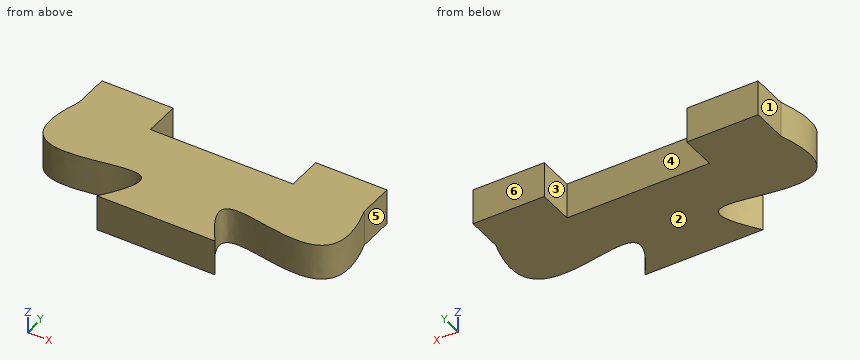
```python
from build123d import *

# Parameters (mm, degrees)
SKETCH1_W           = 6.35
SKETCH1_H           = 3.175
BOSS_EXTRUDE1_DEPTH = 3.175


with BuildPart() as part:
    # Sketch1 → Boss-Extrude1 (new body)
    with BuildSketch(Plane.XY):
        with Locations((-63.39715008, 33.781933128)):
            Rectangle(SKETCH1_W, SKETCH1_H)
        with BuildLine():
            Line((-60.22215008, 32.194433128), (-66.57215008, 32.194433128))
            add(Edge.make_bspline(
                [(-66.57215008, 32.194433128), (-70.796112031, 19.610192525), (-51.766503484, 33.116701814), (-59.124597577, 23.025033128)],
                knots=[0, 0, 0, 0, 1, 1, 1, 1], degree=3))
            Line((-59.124597577, 23.025033128), (-48.619702582, 23.025033128))
            add(Edge.make_bspline(
                [(-41.17215008, 32.194433128), (-36.948188128, 19.610192525), (-55.977796675, 33.116701814), (-48.619702582, 23.025033128)],
                knots=[0, 0, 0, 0, 1, 1, 1, 1], degree=3))
            Line((-41.17215008, 32.194433128), (-47.52215008, 32.194433128))
            Line((-47.52215008, 32.194433128), (-60.22215008, 32.194433128))
        make_face()
        with Locations((-44.34715008, 33.781933128)):
            Rectangle(SKETCH1_W, SKETCH1_H)
    extrude(amount=BOSS_EXTRUDE1_DEPTH)


solid = part.part
```
Can you work these out from the model? Positions are in its coordinate system, mm. Face numbers are marked on the shaded views. A direction names the side the tool comes from. Coordinates: 2 decimals unless noted, no trailing zeros. Loops run counter-clockwise (first coordinate to the right, second up) from the corner with the lowest first, then second, coordinate; pieces in that order, holes last.
1) Imagine slicing it at C-C on y = 27. State how many separate pieces and enclosed holes the cut face has, plus the area to 3 significant figures.
2) Which directions (+Z, -Z, +X, -X, +Y, -Y) give clear straight access to the entire face, cutting with the end or side of a thin tool? Please do the marked faces 1 and 2.
3) For pin 1 (1 mm diameter, centred on y = 34, z = 2, fed in from -X), with a flat end and sliding along its axis, tell me the tip position at first contact or that it passes through.
4) Imagine slicing it at A-A on y = 33.5. List the corners of the cut face in (x, z) for me (3 decimals).
5) Imagine slicing it at B-B on x = -56.25. List the corners of the cut face in (y, z) for me (3 decimals).
6) I need wall thicknesses on probe 1 along X at (y, z) = (33.75, 1.25); probe 2 along X at (y, z) = (29, 2.15); probe 3 along Y at (x, z) = (-54.5, 1.45). Which ranges of each line are inside material? Lowest first, please.
7) Thinking about a two-plate mould opening in X: for the marked faces 3, 4, 5 and 6, which applies, pulls with the +X half, pulls with the -X half, needs draft (parallel to the pull), parting line crosses it, or undercut?
Completed:
1. separate pieces: 3
1. enclosed holes: 0
1. area: 67.8 mm2
2. face 1: +Z, -Z, -X, +Y
2. face 2: -Z, +X, -X, +Y, -Y
3. pin 1: stops at x = -66.57
4. outline: (-66.572, 0) - (-60.222, 0) - (-60.222, 3.175) - (-66.572, 3.175) - close; (-47.522, 0) - (-41.172, 0) - (-41.172, 3.175) - (-47.522, 3.175) - close
5. outline: (23.025, 0) - (32.194, 0) - (32.194, 3.175) - (23.025, 3.175) - close
6. probe 1: x = -66.57 to -60.22, -47.52 to -41.17
6. probe 2: x = -67.19 to -40.55
6. probe 3: y = 23.03 to 32.19
7. face 3: undercut
7. face 4: undercut
7. face 5: pulls with the +X half
7. face 6: needs draft
